```python
from build123d import *
from build123d.topology import SkipClean

# Parameters (mm, degrees)
SALIENTE_EXTRUIR1_DEPTH = 5
CROQUIS2_R              = 2.1
CORTAR_EXTRUIR1_DEPTH   = 83.176639016
CORTAR_EXTRUIR2_DEPTH   = 83.176639016
CROQUIS5_R              = 2.05
CORTAR_EXTRUIR4_DEPTH   = 83.176639016
SALIENTE_EXTRUIR2_DEPTH = 5
CORTAR_EXTRUIR10_DEPTH  = 98.128780493
SALIENTE_EXTRUIR4_DEPTH = 4
SALIENTE_EXTRUIR5_DEPTH = 4
CROQUIS17_R             = 2.4
CORTAR_EXTRUIR11_DEPTH  = 98.128780493
SALIENTE_EXTRUIR6_DEPTH = 104
CORTAR_EXTRUIR12_DEPTH  = 200


with BuildPart() as part:
    # Croquis1 → Saliente-Extruir1 (new body)
    with BuildSketch(Plane(origin=(0, 0, 0), x_dir=(1, 0, 0), z_dir=(0, 1, 0))):
        with BuildLine():
            Line((4, 58), (8.807070745, 49.218243619))
            ThreePointArc((8.807070745, 49.218243619), (35.355339059, 35.355339059), (49.218243619, 8.807070745))
            Line((49.218243619, 8.807070745), (58, 4))
            Line((58, 4), (58, -4))
            Line((58, -4), (49.218243619, -8.807070745))
            ThreePointArc((49.218243619, -8.807070745), (35.355339059, -35.355339059), (8.807070745, -49.218243619))
            Line((8.807070745, -49.218243619), (4, -58))
            Line((4, -58), (-4, -58))
            Line((-4, -58), (-8.807070745, -49.218243619))
            ThreePointArc((-8.807070745, -49.218243619), (-35.355339059, -35.355339059), (-49.218243619, -8.807070745))
            Line((-49.218243619, -8.807070745), (-58, -4))
            Line((-58, -4), (-58, 4))
            Line((-58, 4), (-49.218243619, 8.807070745))
            ThreePointArc((-49.218243619, 8.807070745), (-35.355339059, 35.355339059), (-8.807070745, 49.218243619))
            Line((-8.807070745, 49.218243619), (-4, 58))
            Line((-4, 58), (4, 58))
        make_face()
    extrude(amount=SALIENTE_EXTRUIR1_DEPTH)

    # Croquis2 → Cortar-Extruir1 (cut, through all)
    with BuildSketch(Plane(origin=(0, 5, 0), x_dir=(1, 0, 0), z_dir=(0, 1, 0))):
        with Locations(Location((0, 52.7, 0), (0, 0, 270))):
            Circle(CROQUIS2_R)
        with Locations(Location((52.7, 0, 0), (0, 0, 270))):
            Circle(CROQUIS2_R)
        with Locations(Location((0, -52.7, 0), (0, 0, 270))):
            Circle(CROQUIS2_R)
        with Locations(Location((-52.7, 0, 0), (0, 0, 270))):
            Circle(CROQUIS2_R)
    extrude(amount=-CORTAR_EXTRUIR1_DEPTH, mode=Mode.SUBTRACT)

    # Croquis3 → Cortar-Extruir2 (cut, through all)
    with BuildSketch(Plane(origin=(0, 5, 0), x_dir=(1, 0, 0), z_dir=(0, 1, 0))):
        Polygon((20.506096654, -34.648232278), (34.648232278, -20.506096654), (47.376154339, -33.234018716), (67.218949341, -53.076813717), (53.076813717, -67.218949341), (33.234018716, -47.376154339), align=None)
    extrude(amount=-CORTAR_EXTRUIR2_DEPTH, mode=Mode.SUBTRACT)

    # Croquis5 → Cortar-Extruir4 (cut, through all)
    with BuildSketch(Plane(origin=(0, 5, 0), x_dir=(1, 0, 0), z_dir=(0, 1, 0))):
        with Locations(Location((-7.78, 7.78, 0), (0, 0, 270))):
            Circle(CROQUIS5_R)
        with Locations(Location((7.78, 7.78, 0), (0, 0, 270))):
            Circle(CROQUIS5_R)
        with Locations(Location((7.78, -7.78, 0), (0, 0, 270))):
            Circle(CROQUIS5_R)
        with Locations(Location((-7.78, -7.78, 0), (0, 0, 270))):
            Circle(CROQUIS5_R)
        with BuildLine():
            Line((21.554064831, -30.039346205), (23.334523779, -31.819805153))
            Line((23.334523779, -31.819805153), (24.748737342, -30.405591591))
            Line((24.748737342, -30.405591591), (22.968278393, -28.625132642))
            ThreePointArc((22.968278393, -28.625132642), (19.622213178, -26.69328099), (21.554064831, -30.039346205))
        make_face()
        with BuildLine():
            Line((28.625132642, -22.968278393), (30.986174209, -25.329319959))
            Line((30.986174209, -25.329319959), (32.400387771, -23.915106397))
            Line((32.400387771, -23.915106397), (30.039346205, -21.554064831))
            ThreePointArc((30.039346205, -21.554064831), (26.69328099, -19.622213178), (28.625132642, -22.968278393))
        make_face()
    extrude(amount=-CORTAR_EXTRUIR4_DEPTH, mode=Mode.SUBTRACT)

    # Croquis7 → Saliente-Extruir2 (add, through all)
    with BuildSketch(Plane(origin=(0, 5, 0), x_dir=(1, 0, 0), z_dir=(0, 1, 0))):
        Polygon((68.589357775, -54.447222151), (54.447222151, -68.589357775), (8.807070745, -49.218243619), (18.571685103, -46.422973972), (27.56994834, -41.712083963), (48.790367902, -62.932503526), (62.932503526, -48.790367902), (41.712083963, -27.56994834), (46.422973972, -18.571685103), (49.218243619, -8.807070745), align=None)
    extrude(amount=-SALIENTE_EXTRUIR2_DEPTH)

    # Croquis8 → Cortar-Extruir10 (cut, through all)
    with BuildSketch(Plane(origin=(0, 5, 0), x_dir=(1, 0, 0), z_dir=(0, 1, 0))):
        with BuildLine():
            Line((54.283137452, -59.939991701), (51.490214314, -57.147068564))
            Line((51.490214314, -57.147068564), (50.076000752, -58.561282126))
            Line((50.076000752, -58.561282126), (52.868923889, -61.354205264))
            ThreePointArc((52.868923889, -61.354205264), (56.214989104, -63.286056916), (54.283137452, -59.939991701))
        make_face()
        with BuildLine():
            Line((57.371843354, -51.714989104), (58.786056916, -50.300775542))
            Line((58.786056916, -50.300775542), (61.354205264, -52.868923889))
            ThreePointArc((61.354205264, -52.868923889), (63.286056916, -56.214989104), (59.939991701, -54.283137452))
            Line((59.939991701, -54.283137452), (57.371843354, -51.714989104))
        make_face()
    extrude(amount=-CORTAR_EXTRUIR10_DEPTH, mode=Mode.SUBTRACT)

    # Croquis15 → Saliente-Extruir4 (add)
    with BuildSketch(Plane.XZ):
        with BuildLine():
            Line((-1.111111111, -20.469866441), (-1.111111111, -22.472548411))
            ThreePointArc((-1.111111111, -22.472548411), (0, 22.5), (1.111111111, -22.472548411))
            Line((1.111111111, -22.472548411), (1.111111111, -20.469866441))
            ThreePointArc((1.111111111, -20.469866441), (0, 20.5), (-1.111111111, -20.469866441))
        make_face()
    extrude(amount=SALIENTE_EXTRUIR4_DEPTH)

    # Croquis16 → Saliente-Extruir5 (add)
    with SkipClean():  # the faces are left unmerged after this step: merging them gives an invalid solid
        with BuildSketch(Plane.XZ):
            with BuildLine():
                Line((-1.111111111, -20.469866441), (-1.111111111, -22.472548411))
                ThreePointArc((-1.111111111, -22.472548411), (0, -22.5), (1.111111111, -22.472548411))
                Line((1.111111111, -22.472548411), (1.111111111, -20.469866441))
                ThreePointArc((1.111111111, -20.469866441), (0, -20.5), (-1.111111111, -20.469866441))
            make_face()
        extrude(amount=SALIENTE_EXTRUIR5_DEPTH)

    # Croquis17 → Cortar-Extruir11 (cut, through all)
    with SkipClean():  # the faces are left unmerged after this step: merging them gives an invalid solid
        with BuildSketch(Plane.XZ):
            with Locations(Location((42.43, 0, 0), (0, 0, 270))):
                Circle(CROQUIS17_R)
            with Locations(Location((0, -42.43, 0), (0, 0, 270))):
                Circle(CROQUIS17_R)
            with Locations(Location((-42.43, 0, 0), (0, 0, 270))):
                Circle(CROQUIS17_R)
            with Locations(Location((0, 42.43, 0), (0, 0, 270))):
                Circle(CROQUIS17_R)
        extrude(amount=-CORTAR_EXTRUIR11_DEPTH, mode=Mode.SUBTRACT)

    # Croquis18 → Saliente-Extruir6 (add)
    with SkipClean():  # the faces are left unmerged after this step: merging them gives an invalid solid
        with BuildSketch(Plane(origin=(0, 5, 0), x_dir=(1, 0, 0), z_dir=(0, 1, 0))):
            with BuildLine():
                Line((-7.026199157, 59.180786921), (-10.712769702, 52.416472271))
                ThreePointArc((-10.712769702, 52.416472271), (-37.80704006, 37.853371341), (-52.403312858, 10.776956969))
                Line((-52.403312858, 10.776956969), (-59.137075713, 7.002717611))
                Line((-59.137075713, 7.002717611), (-61.456288791, 5.738739948))
                Line((-61.456288791, 5.738739948), (-61.456288791, -5.78570304))
                Line((-61.456288791, -5.78570304), (-59.137075713, -7.049680703))
                Line((-59.137075713, -7.049680703), (-52.416550741, -10.71238575))
                ThreePointArc((-52.416550741, -10.71238575), (-37.841055246, -37.819367233), (-10.74243433, -52.41040073))
                Line((-10.74243433, -52.41040073), (-6.959006403, -59.160557259))
                Line((-6.959006403, -59.160557259), (-5.695028739, -61.479770337))
                Line((-5.695028739, -61.479770337), (5.829414249, -61.479770337))
                Line((5.829414249, -61.479770337), (7.093391912, -59.160557259))
                Line((7.093391912, -59.160557259), (10.133049539, -53.583232651))
                Line((10.133049539, -53.583232651), (55.252838681, -72.733488714))
                Line((55.252838681, -72.733488714), (72.733488714, -55.252838681))
                Line((72.733488714, -55.252838681), (53.583232651, -10.133049539))
                Line((53.583232651, -10.133049539), (59.204268467, -6.982487949))
                Line((59.204268467, -6.982487949), (61.523481546, -5.718510285))
                Line((61.523481546, -5.718510285), (61.523481546, 5.805932703))
                Line((61.523481546, 5.805932703), (59.204268467, 7.069910366))
                Line((59.204268467, 7.069910366), (52.403430197, 10.776386386))
                ThreePointArc((52.403430197, 10.776386386), (37.849997802, 37.810417433), (10.831208274, 52.392126578))
                Line((10.831208274, 52.392126578), (7.026199157, 59.180786921))
                Line((7.026199157, 59.180786921), (5.762221494, 61.5))
                Line((5.762221494, 61.5), (-5.762221494, 61.5))
                Line((-5.762221494, 61.5), (-7.026199157, 59.180786921))
            make_face()
        extrude(amount=SALIENTE_EXTRUIR6_DEPTH)

    # Croquis23 → Cortar-Extruir12 (cut)
    with BuildSketch(Plane.XZ.offset(4)):
        with BuildLine():
            Line((59, -4.59262422), (58.95889986, -4.615122143))
            Line((58.95889986, -4.615122143), (50.492416575, -9.249614646))
            ThreePointArc((50.492416575, -9.249614646), (36.297654901, -36.297654901), (9.249614646, -50.492416575))
            Line((9.249614646, -50.492416575), (4.615122143, -58.95889986))
            Line((4.615122143, -58.95889986), (4.592624221, -59))
            Line((4.592624221, -59), (-4.59262422, -59))
            Line((-4.59262422, -59), (-4.615122143, -58.95889986))
            Line((-4.615122143, -58.95889986), (-9.249614646, -50.492416575))
            ThreePointArc((-9.249614646, -50.492416575), (-36.297654901, -36.297654901), (-50.492416575, -9.249614646))
            Line((-50.492416575, -9.249614646), (-58.95889986, -4.615122143))
            Line((-58.95889986, -4.615122143), (-59, -4.592624221))
            Line((-59, -4.592624221), (-59, 4.59262422))
            Line((-59, 4.59262422), (-58.95889986, 4.615122143))
            Line((-58.95889986, 4.615122143), (-50.492416575, 9.249614646))
            ThreePointArc((-50.492416575, 9.249614646), (-36.297654901, 36.297654901), (-9.249614646, 50.492416575))
            Line((-9.249614646, 50.492416575), (-4.615122143, 58.95889986))
            Line((-4.615122143, 58.95889986), (-4.592624221, 59))
            Line((-4.592624221, 59), (4.59262422, 59))
            Line((4.59262422, 59), (4.615122143, 58.95889986))
            Line((4.615122143, 58.95889986), (9.249614646, 50.492416575))
            Line((9.249614646, 50.492416575), (54.677398303, 69.773395186))
            Line((54.677398303, 69.773395186), (69.773395186, 54.677398303))
            Line((69.773395186, 54.677398303), (50.492416575, 9.249614646))
            Line((50.492416575, 9.249614646), (58.95889986, 4.615122143))
            Line((58.95889986, 4.615122143), (59, 4.592624221))
            Line((59, 4.592624221), (59, -4.59262422))
        make_face()
    extrude(amount=-CORTAR_EXTRUIR12_DEPTH, mode=Mode.SUBTRACT)


solid = part.part
```
Could you check a few things on this model? Use its own coordinates, in mm. A direction names the side the tool comes from. Give positions to 0.01 mm unless a question says otherwise; leave off trailing zeros. Order: outer loops, then holes, each group sorted by start corner. A loop starts at its lowest first (then second) coordinate and runs counter-clockwise, first axis right, second up.
Q1. Suppose I cut it at B-B, the plane x = 32.5. Write out the boundary of the cut face in (y, z).
Q2. I'm going to push flat-ended pins straight in: P1, Ø8, axis at y = 74, z = -12.5, coming from the -X side; P2, Ø10, axis at x = 18, y = 76.5, coming from the -Z side; P3, Ø10, axis at x = 48.5, z = 3.5, coming from the -Y side; P4, Ø1.5, axis at x = -31, y = 64.5, coming from the +Z side. Where does each tip first touch, or does it pass through?
Q3. If I drill on line 1 along Z through (x, y) = (2, 33); line 2 along Z through (x, y) = (60, 70); line 3 along Z through (x, y) = (16, 80.5), over which ranges is the centre line in solid material (lowest first)?
Q4. Suppose I cut it at A-A, the plane z = 2.5. Write out the boundary of the cut face in (x, y), and give its area (3 significant figures).
Q5. For faces 1 (the flat face through (-59, 56, 0)), 2 (the flat face through (61.523, 56, 0)), 3 (the flat face through (32.377, 56.272, 63.024)), which set-ups out of +Z, -Z, +X, -X, +Y, -Y let a thin tool reach every point of the face, with its end or its side?
Solution:
1. outline: (5, -42.5) - (109, -42.5) - (109, -39.73) - (5, -39.73) - close; (5, 60.36) - (109, 60.36) - (109, 63.08) - (5, 63.08) - close
2. P1: stops at x = -56.47
2. P2: stops at z = -51.9
2. P3: passes through
2. P4: stops at z = 44.13
3. line 1: z = -61.5 to -59, 59 to 61.48
3. line 2: z = -6.64 to 6.55, 25.25 to 31.65, 64.45 to 67.99
3. line 3: z = -51.05 to -48.78, 53.36 to 56.07
4. outline: (-61.46, 5) - (-59, 5) - (-59, 109) - (-61.46, 109) - close; (59, 5) - (61.52, 5) - (61.52, 109) - (59, 109) - close
4. area: 518 mm2
5. face 1: +Y, -Y
5. face 2: -Z, +X, +Y, -Y
5. face 3: +Z, +Y, -Y
